Read the model definition and answer for the solid it produces. Units are mm, in the model's axes. A direction names the side the tool comes from. Give positions to 0.01 mm unless a question says otherwise; leave off trailing zeros. Order: outer loops, then holes, each group sorted by start corner. A loop starts at its lowest first (then second) coordinate and runs counter-clockwise, first axis right, second up. Notation, with made-up numbers: (46.5, 23.5) -> (55.5, 23.5) arc R18 cw to (55.5, 39.5) -> close; hole circle Ø2 at (50.25, -23). An arc over 180 degrees is marked (long way). One line per item, written item: value. Start each with the question number.
from build123d import *

# Parameters (mm, degrees)
BOSS_EXTRUDE1_DEPTH = 0.0001
BOSS_EXTRUDE2_DEPTH = 2
BOSS_EXTRUDE3_DEPTH = 0.0001
SKETCH4_R           = 8
BOSS_EXTRUDE4_DEPTH = 9.5
SKETCH5_R           = 6.5
CUT_EXTRUDE1_DEPTH  = 25
CUT_EXTRUDE4_DEPTH  = 7.5
CIRPATTERN2_COUNT   = 4


with BuildPart() as part:
    # Sketch1 → Boss-Extrude1 (new body)
    with BuildSketch(Plane.XY):
        with BuildLine():
            Line((-5.05, 9.000108401), (5.05, 9.000108401))
            ThreePointArc((5.05, 9.000108401), (7.878427125, 7.828535526), (9.05, 5.000108401))
            Line((9.05, 5.000108401), (9.05, -5.000108401))
            ThreePointArc((9.05, -5.000108401), (7.878427125, -7.828535526), (5.05, -9.000108401))
            Line((5.05, -9.000108401), (-5.05, -9.000108401))
            ThreePointArc((-5.05, -9.000108401), (-7.878427125, -7.828535526), (-9.05, -5.000108401))
            Line((-9.05, -5.000108401), (-9.05, 5.000108401))
            ThreePointArc((-9.05, 5.000108401), (-7.878427125, 7.828535526), (-5.05, 9.000108401))
        make_face()
    extrude(amount=BOSS_EXTRUDE1_DEPTH)

    # Sketch2 → Boss-Extrude2 (add)
    with BuildSketch(Plane.XY):
        with BuildLine():
            Line((-5.05, 9.000108401), (5.05, 9.000108401))
            ThreePointArc((5.05, 9.000108401), (7.878427125, 7.828535526), (9.05, 5.000108401))
            Line((9.05, 5.000108401), (9.05, -5.000108401))
            ThreePointArc((9.05, -5.000108401), (7.878427125, -7.828535526), (5.05, -9.000108401))
            Line((5.05, -9.000108401), (-5.05, -9.000108401))
            ThreePointArc((-5.05, -9.000108401), (-7.878427125, -7.828535526), (-9.05, -5.000108401))
            Line((-9.05, -5.000108401), (-9.05, 5.000108401))
            ThreePointArc((-9.05, 5.000108401), (-7.878427125, 7.828535526), (-5.05, 9.000108401))
        make_face()
    extrude(amount=BOSS_EXTRUDE2_DEPTH)

    # Sketch3 → Boss-Extrude3 (add)
    with BuildSketch(Plane.XY.offset(2)):
        with BuildLine():
            Line((-5.05, 9.000108401), (5.05, 9.000108401))
            ThreePointArc((5.05, 9.000108401), (7.878427125, 7.828535526), (9.05, 5.000108401))
            Line((9.05, 5.000108401), (9.05, -5.000108401))
            ThreePointArc((9.05, -5.000108401), (7.878427125, -7.828535526), (5.05, -9.000108401))
            Line((5.05, -9.000108401), (-5.05, -9.000108401))
            ThreePointArc((-5.05, -9.000108401), (-7.878427125, -7.828535526), (-9.05, -5.000108401))
            Line((-9.05, -5.000108401), (-9.05, 5.000108401))
            ThreePointArc((-9.05, 5.000108401), (-7.878427125, 7.828535526), (-5.05, 9.000108401))
        make_face()
    extrude(amount=BOSS_EXTRUDE3_DEPTH)

    # Sketch4 → Boss-Extrude4 (add)
    with BuildSketch(Plane.XY.offset(2.0001)):
        Circle(SKETCH4_R)
    extrude(amount=BOSS_EXTRUDE4_DEPTH)

    # Sketch5 → Cut-Extrude1 (cut, symmetric)
    with BuildSketch(Plane.XY.offset(2.0001)):
        Circle(SKETCH5_R)
    extrude(amount=CUT_EXTRUDE1_DEPTH, both=True, mode=Mode.SUBTRACT)

    # Sketch15 → Cut-Extrude4 (cut)
    with BuildSketch(Plane.XY.offset(11.5001)):
        Polygon((-0.552830798, 8.187091014), (-0.002830798, 0.003314653), (0.547169202, 8.187091014), (0.617169202, 9.000108401), (-0.626042329, 9.000108401), align=None)
    cut_extrude4 = extrude(amount=-CUT_EXTRUDE4_DEPTH, mode=Mode.SUBTRACT)

    # CirPattern2: Cut-Extrude4 ×4 about axis
    cirpattern2_axis = Axis((0, 0, 0), (0, 0, 1))
    for i in range(1, CIRPATTERN2_COUNT):
        add(cut_extrude4.rotate(cirpattern2_axis, i * 360 / CIRPATTERN2_COUNT), mode=Mode.SUBTRACT)


solid = part.part
Item 1: Find section D-D on z = 3.75. Write down the section's boundary in (x, y), then the cut area to 3 significant figures.
Item 2: Find section B-B on y = 0. Write down the section's boundary in (x, z).
Item 3: Find section C-C on x = 0. Write down the section's boundary in (y, z), then the cut area to 3 significant figures.
Item 4: Flat-ended cylindrical pins translate along their axes: pin 1 (1 mm diameter, centred on x = 3.5, z = 4.5, fed in from +Y); pin 2 (6 mm diameter, centred on x = 0, z = 9, fed in from +Y). Find the tip coordinate at first contact, or state that the pin passes through.
Item 5: Find the intervals of material crossed by line 1 (X direction, y = 0, z = 2.75); line 2 (Z direction, x = 7, y = 6); line 3 (Y direction, x = 0.75, z = 4.5), in increasing order. Write a range as from..to.
Item 6: Find section A-A on z = 9.5. Write down the section's boundary in (x, y).
Item 7: A tool of negligible diameter and unlimited length cuts with its end or side. For faces 4 (the flat face through (0.49, -7.24, 7.8)), 5 (the cylindrical face through (7.39, -3.06, 6.68)), 6 (the flat face through (0, 7, 4)), 7 (the flat face through (-7, 0, 4)), from which of +Z, -Z, +X, -X, +Y, -Y can it reach the whole face along a straight path? Write none if from no direction.
Item 8: For a pull along Y with two mould halves and no side action, classify faces 1 (the cylindrical face through (-7.847, -7.859, 0.986)), 2 (the flat face through (-0.49, 7.24, 7.8)), 3 (the flat face through (7.24, 0.49, 7.8)) as +Y half, -Y half, draft (parallel to the pull), parting line (faces both ways), or undercut.
Checks:
1. outline: circle Ø16 at (0, 0); hole circle Ø13 at (0, 0)
1. area: 68.3 mm2
2. outline: (-9.05, 0) -> (-6.5, 0) -> (-6.5, 4) -> (-8, 4) -> (-8, 2) -> (-9.05, 2) -> close; (6.5, 0) -> (9.05, 0) -> (9.05, 2) -> (8, 2) -> (8, 4) -> (6.5, 4) -> close
3. outline: (-9, 0) -> (-6.5, 0) -> (-6.5, 4) -> (-8, 4) -> (-8, 2) -> (-9, 2) -> close; (6.5, 0) -> (9, 0) -> (9, 2) -> (8, 2) -> (8, 4) -> (6.5, 4) -> close
3. area: 16.0 mm2
4. pin 1: y = 7.42
4. pin 2: y = 7.98
5. line 1: -8..-6.5, 6.5..8
5. line 2: 0..2
5. line 3: -7.96..-6.46, 6.46..7.96
6. outline: (-7.98, -0.54) arc R8 ccw to (-0.53, -7.98) -> (-0.43, -6.49) arc R6.5 cw to (-6.49, -0.44) -> close; (-7.98, 0.53) -> (-6.49, 0.43) arc R6.5 cw to (-0.44, 6.49) -> (-0.54, 7.98) arc R8 ccw to start; (0.43, 6.49) arc R6.5 cw to (6.49, 0.44) -> (7.98, 0.54) arc R8 ccw to (0.53, 7.98) -> close; (0.44, -6.49) -> (0.54, -7.98) arc R8 ccw to (7.98, -0.53) -> (6.49, -0.43) arc R6.5 cw to start
7. face 4: +Z, -Y
7. face 5: +Z
7. face 6: +Z, +Y
7. face 7: +Z, -X
8. face 1: -Y half
8. face 2: +Y half
8. face 3: undercut
